Geometry: see drawing. Coordinates: mm, zero at the bounding-box minimum. A direction names the side the tool comes from. Coordinates: 2 decimals unless noted, no trailing zeros. Loops run counter-clockwise (first coordinate to the right, second up) from the corner with the lowest first, then second, coordinate; pieces in that order, holes last.
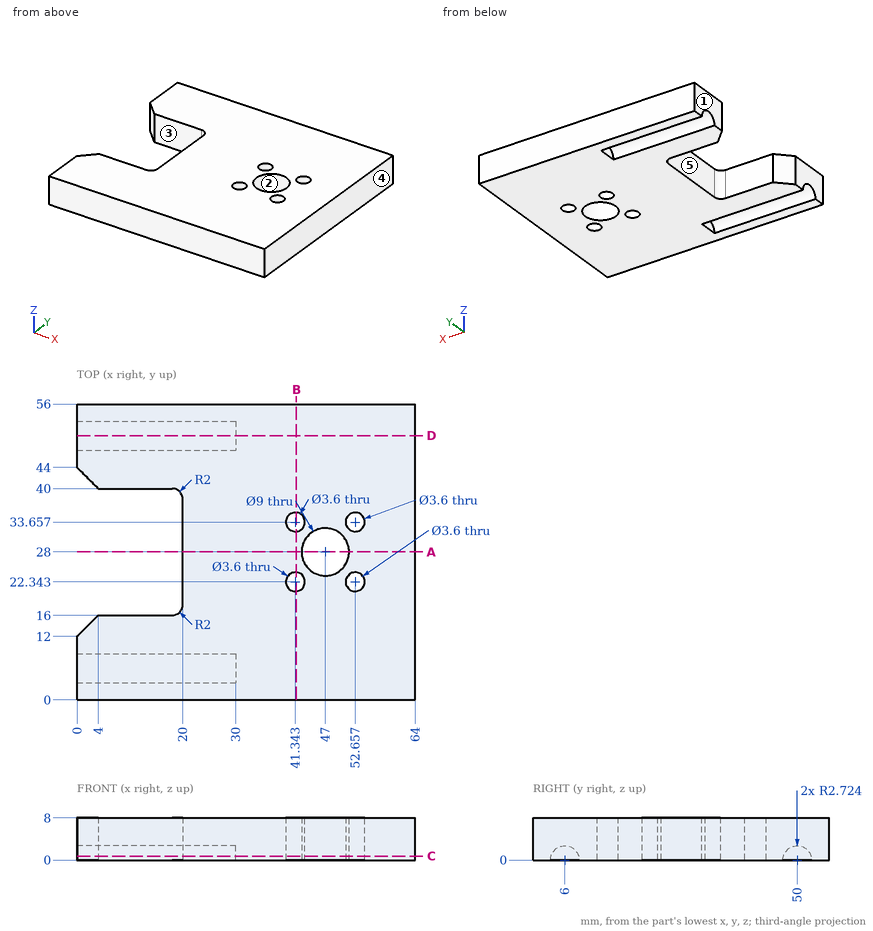
Item 1: Line query: L1, parallel to Y at x = 13.5, z = 1; L2, parallel to X at y = 21.5, z = 2.5; L3, parallel to Y at x = 7, z = 5.5. Output: solid intervals per line, ascending.
Result:
L1: y = 0 to 3.47, 8.53 to 16, 40 to 47.47, 52.53 to 56
L2: x = 20 to 39.75, 42.93 to 51.07, 54.25 to 64
L3: y = 0 to 16, 40 to 56
Item 2: Section query A-A (y = 28). Output: boundary loops of the cut face in (x, z), then the cut area to 3 significant figures.
Result:
outline: (20, 0) - (42.5, 0) - (42.5, 8) - (20, 8) - close; (51.5, 0) - (64, 0) - (64, 8) - (51.5, 8) - close
area: 280 mm2
Item 3: Reachability of the marked faces 4 and 5 from +Z, -Z, +X, -X, +Y, -Y: full face, straight path, thin tool, end or side. Return the list, or none.
Result:
face 4: +Z, -Z, +X, +Y, -Y
face 5: +Z, -Z, -X
Item 4: Section query C-C (z = 0.75). Output: boundary loops of the cut face in (x, y).
Result:
outline: (0, 0) - (64, 0) - (64, 56) - (0, 56) - (0, 52.62) - (30, 52.62) - (30, 47.38) - (0, 47.38) - (0, 44) - (4, 40) - (18, 40) arc R2 cw to (20, 38) - (20, 18) arc R2 cw to (18, 16) - (4, 16) - (0, 12) - (0, 8.62) - (30, 8.62) - (30, 3.38) - (0, 3.38) - close; hole circle Ø3.6 at (41.34, 22.34); hole circle Ø3.6 at (41.34, 33.66); hole circle Ø9 at (47, 28); hole circle Ø3.6 at (52.66, 22.34); hole circle Ø3.6 at (52.66, 33.66)
Item 5: Section query D-D (y = 50). Output: boundary loops of the cut face in (x, z), then the cut area to 3 significant figures.
Result:
outline: (0, 2.72) - (30, 2.72) - (30, 0) - (64, 0) - (64, 8) - (0, 8) - close
area: 430 mm2
Item 6: Section query B-B (x = 41.5). Output: boundary loops of the cut face in (y, z), then the cut area to 3 significant figures.
Result:
outline: (0, 0) - (20.55, 0) - (20.55, 8) - (0, 8) - close; (24.14, 0) - (31.86, 0) - (31.86, 8) - (24.14, 8) - close; (35.45, 0) - (56, 0) - (56, 8) - (35.45, 8) - close
area: 391 mm2
Item 7: Mould query, pull axis X, two halves, no side actions, for the marked faces 1, 2 and 3. Classes: +X half, -X half, draft (parallel to the pull), parting line (faces both ways), or undercut.
Result:
face 1: -X half
face 2: undercut
face 3: draft
Item 8: Contact query for flat-ended pins moving along their axis: P1, Ø6, axis at x = 41.34, y = 22.34, coming from the -Z side; P2, Ø1.4, axis at y = 49, z = 1.5, coming from the -X side. Output: stop coordinate, or through.
Result:
P1: stops at z = 0
P2: stops at x = 30
